Could you check a few things on this drawing? It's one solid part, dimensions in mm from its lowest x, y, z. A direction names the side the tool comes from. Give positions to 0.01 mm unless a question says otherwise; leave off trailing zeros. Order: outer loops, then holes, each group sorted by start corner. A loop starts at its lowest first (then second) coordinate and runs counter-clockwise, first axis right, second up.
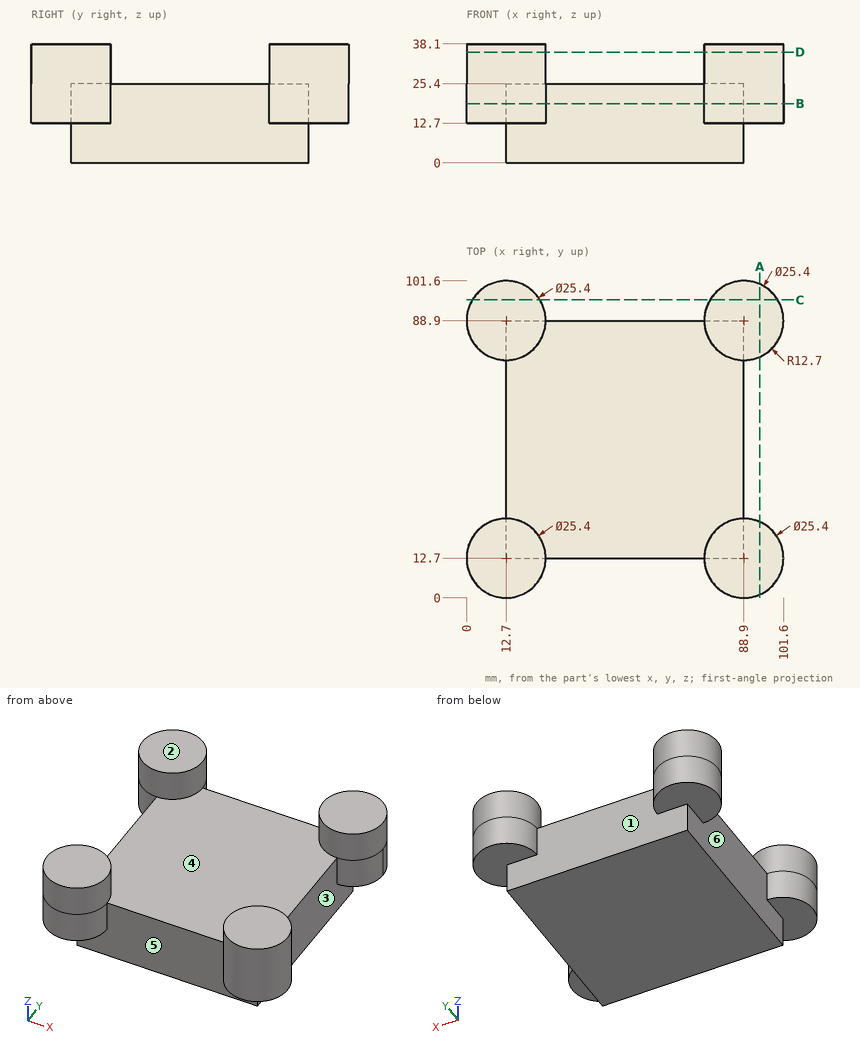
Q1. I need wall thicknesses on L1, parallel to Y at x = 12.5, z = 27.5; L2, parallel to X at y = 12, z = 15.5; L3, parallel to Y at x = 61, z = 3. Which ranges of each line are inside material? Lowest first, please.
Filled sheet:
L1: y = 0 to 25.4, 76.2 to 101.6
L2: x = 0.02 to 25.38, 76.22 to 101.58
L3: y = 12.7 to 88.9
Q2. If we section it at A-A on x = 94: List the corners of the cut face in (y, z) for me.
Filled sheet:
outline: (1.07, 12.7) - (24.33, 12.7) - (24.33, 38.1) - (1.07, 38.1) - close; (77.27, 12.7) - (100.53, 12.7) - (100.53, 38.1) - (77.27, 38.1) - close
Q3. If we section it at D-D on z = 35.5: List the corners of the cut face in (x, y) for me, plus the area to 3 significant figures.
Filled sheet:
outline: circle Ø25.4 at (12.7, 12.7); circle Ø25.4 at (12.7, 88.9); circle Ø25.4 at (88.9, 12.7); circle Ø25.4 at (88.9, 88.9)
area: 2,030 mm2
Q4. If we section it at C-C on y = 95.5: List the corners of the cut face in (x, z) for me, plus the area to 3 significant figures.
Filled sheet:
outline: (1.85, 12.7) - (23.55, 12.7) - (23.55, 38.1) - (1.85, 38.1) - close; (78.05, 12.7) - (99.75, 12.7) - (99.75, 38.1) - (78.05, 38.1) - close
area: 1,100 mm2
Q5. If we section it at B-B on z = 19: List the corners of the cut face in (x, y) for me.
Filled sheet:
outline: (12.7, 25.4) arc R12.7 ccw (long way) to (25.4, 12.7) - (76.2, 12.7) arc R12.7 ccw (long way) to (88.9, 25.4) - (88.9, 76.2) arc R12.7 ccw (long way) to (76.2, 88.9) - (25.4, 88.9) arc R12.7 ccw (long way) to (12.7, 76.2) - close
Q6. Thinking about a two-plate mould opening in Y: for the marked faces 1, 2 and 3, which applies, released by +Y, released by -Y, zero draft, split by the parting line, or undercut?
Filled sheet:
face 1: released by +Y
face 2: zero draft
face 3: undercut
Q7. For the marked faces 4, 5 and 6, which set-ups out of +Z, -Z, +X, -X, +Y, -Y let a thin tool reach every point of the face, with its end or its side?
Filled sheet:
face 4: +Z
face 5: -Z, -Y
face 6: -Z, -X
Q8. I'm going to push flat-ended pins straight in: P1, Ø12.5, axis at x = 37.5, z = 7, coming from the -Y side; P2, Ø1.5, axis at y = 24.5, z = 4.5, coming from the +X side; P3, Ø7.5, axis at y = 40, z = 15, coming from the -X side. Where does each tip first touch, or does it pass through?
Filled sheet:
P1: stops at y = 12.7
P2: stops at x = 88.9
P3: stops at x = 12.7
